from build123d import *

# Parameters (mm, degrees)
SKETCH1_R           = 44.45
SKETCH1_R_2         = 19.05
SKETCH1_R_3         = 1.410622882
SKETCH1_R_4         = 1.22190068
SKETCH1_R_5         = 0.971343814
BOSS_EXTRUDE1_DEPTH = 5.08
BOSS_EXTRUDE2_DEPTH = 5.08
SKETCH3_W           = 88.9
SKETCH3_H           = 5.08
EXTRUDE_THIN1_DEPTH = 76.2
BOSS_EXTRUDE3_DEPTH = 5.08


with BuildPart() as part:
    # Sketch1 → Boss-Extrude1 (new body)
    with BuildSketch(Plane(origin=(0, 0, 0), x_dir=(1, 0, 0), z_dir=(0, 1, 0))):
        with Locations(Location((0, 0, 0), (0, 0, 270))):
            Circle(SKETCH1_R)
        with Locations(Location((0, 0, 0), (0, 0, 270))):
            Circle(SKETCH1_R_2, mode=Mode.SUBTRACT)
        with Locations(Location((0, 25.4, 0), (0, 0, 270))):
            Circle(SKETCH1_R_3, mode=Mode.SUBTRACT)
        with Locations(Location((21.997045256, -12.7, 0), (0, 0, 270))):
            Circle(SKETCH1_R_4, mode=Mode.SUBTRACT)
        with Locations(Location((-21.997045256, -12.7, 0), (0, 0, 270))):
            Circle(SKETCH1_R_5, mode=Mode.SUBTRACT)
    extrude(amount=BOSS_EXTRUDE1_DEPTH)

    # Sketch2 → Boss-Extrude2 (add)
    with BuildSketch(Plane(origin=(0, 0, 0), x_dir=(1, 0, 0), z_dir=(0, 1, 0))):
        with BuildLine():
            Line((-44.45, 0), (-44.45, -50.8))
            Line((-44.45, -50.8), (44.45, -50.8))
            Line((44.45, -50.8), (44.45, 0))
            ThreePointArc((44.45, 0), (0, -44.45), (-44.45, 0))
        make_face()
    extrude(amount=BOSS_EXTRUDE2_DEPTH)

    # Sketch3 → Extrude-Thin1 (add)
    with BuildSketch(Plane(origin=(0, 5.08, 0), x_dir=(1, 0, 0), z_dir=(0, 1, 0))):
        with Locations((0, -48.26)):
            Rectangle(SKETCH3_W, SKETCH3_H)
    extrude(amount=EXTRUDE_THIN1_DEPTH)

    # Sketch4 → Boss-Extrude3 (add)
    with BuildSketch(Plane.ZY.offset(44.45)):
        Polygon((0, 5.08), (0, 17.78), (33.02, 81.28), (45.72, 81.28), (45.72, 5.08), align=None)
    boss_extrude3 = extrude(amount=-BOSS_EXTRUDE3_DEPTH)

    # Mirror1: Boss-Extrude3 across plane
    add(boss_extrude3.mirror(Plane(origin=(0, 0, 0), x_dir=(0, 0, 1), z_dir=(1, 0, 0))))


solid = part.part
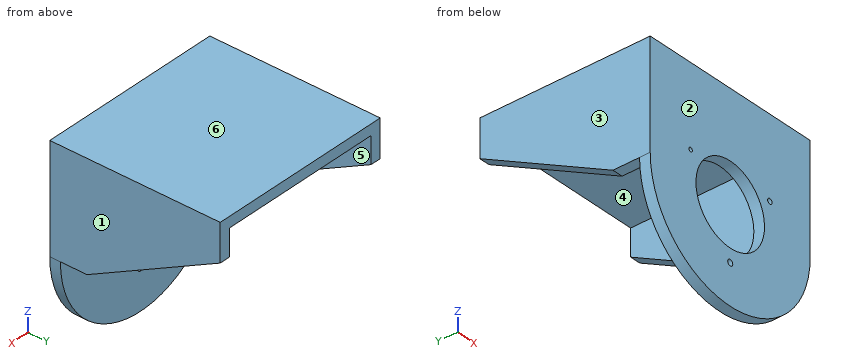
Geometry: final body of the model. Coordinates: model frame, mm. Face numbers are marked on the shaded views. A direction names the side the tool comes from. Round coordinates to 2 decimals unless told otherwise and drop trailing zeros. Order: outer loops, then holes, each group sorted by start corner. A loop starts at its lowest first (then second) coordinate and runs counter-clockwise, first axis right, second up. Notation, with made-up numbers: (65.25, 51) -> (92.25, 51) arc R30 ccw to (92.25, 80) -> close; hole circle Ø9 at (59, 24). An arc over 180 degrees is marked (long way). Put each result on its own line as item: value. Start each with the question number.
Q1. Pull-direction query (X, two-part tool) for the marked faces 1, 2, 3 and 4; classes: +X half, -X half, draft (parallel to the pull), parting line (faces both ways), or undercut.
Q2. Reachability of the marked faces 5 and 6 from +Z, -Z, +X, -X, +Y, -Y: full face, straight path, thin tool, end or side. Return the list, or none.
Q3. Section A-A on x = 0. Return the cut outline in (y, z).
Q4. Section C-C on y = 47.5. Return the cut outline in (x, z).
Q5. First-contact query: pin 1 (23 mm diameter, centred on x = -3, y = 34.5, fed in from -Z); pin 2 (1.5 mm diameter, centred on x = 42.5, y = 13.5, fed in from -Z); pin 3 (3.5 mm diameter, centred on x = 0, z = -25.4, fed in from -Y); pin 4 (5 mm diameter, centred on x = -4.5, z = -25, fed in from +Y). Flat tips, straight axial feed; report the tip coordinate or a pass-through.
Q6. Line query: probe 1 along X at (y, z) = (2, 12); probe 2 along X at (y, z) = (3.4, 12.7); probe 3 along X at (y, z) = (66, 33). Output: solid intervals per line, ascending.
Q7. Section D-D on z = -25.4. Return the cut outline in (x, y), and give its area (3 significant figures).
Q8. Section B-B on x = 10. Return the cut outline in (y, z).
Ans:
1. face 1: +X half
1. face 2: draft
1. face 3: -X half
1. face 4: undercut
2. face 5: -Z, +Y
2. face 6: +Z, +X, -X, +Y, -Y
3. outline: (0, -44.45) -> (5.08, -44.45) -> (5.08, -26.81) -> (0, -26.81) -> close; (0, -23.99) -> (5.08, -23.99) -> (5.08, -19.05) -> (0, -19.05) -> close; (0, 19.05) -> (5.08, 19.05) -> (5.08, 45.72) -> (81.28, 45.72) -> (81.28, 50.8) -> (0, 50.8) -> close
4. outline: (-44.45, 15.45) -> (-39.37, 15.45) -> (-39.37, 45.72) -> (39.37, 45.72) -> (39.37, 15.45) -> (44.45, 15.45) -> (44.45, 50.8) -> (-44.45, 50.8) -> close
5. pin 1: stops at z = 45.72
5. pin 2: stops at z = 0
5. pin 3: stops at y = 0
5. pin 4: stops at y = 5.08
6. probe 1: x = -44.45 to -22.67, -21.32 to -14.8, 14.8 to 21, 23 to 44.45
6. probe 2: x = -44.45 to -22.97, -21.03 to -14.2, 14.2 to 20.78, 23.22 to 44.45
6. probe 3: x = -44.45 to -39.37, 39.37 to 44.45
7. outline: (-36.48, 0) -> (-1.41, 0) -> (-1.41, 5.08) -> (-36.48, 5.08) -> close; (1.41, 0) -> (36.48, 0) -> (36.48, 5.08) -> (1.41, 5.08) -> close
7. area: 356 mm2
8. outline: (0, -43.31) -> (5.08, -43.31) -> (5.08, -16.21) -> (0, -16.21) -> close; (0, 16.21) -> (5.08, 16.21) -> (5.08, 45.72) -> (81.28, 45.72) -> (81.28, 50.8) -> (0, 50.8) -> close
